```python
from build123d import *

# Parameters (mm, degrees)
BOSS_EXTRU_1_DEPTH      = 5.5
ESQUISSE6_W             = 12
ESQUISSE6_H             = 12
BOSS_EXTRU_4_DEPTH      = 4
ESQUISSE7_R             = 1.75
BOSS_EXTRU_7_DEPTH      = 0.5
ESQUISSE8_R             = 1.5
BOSS_EXTRU_9_DEPTH      = 5
CONG_1_R                = 1
CONG_2_R                = 1
CONG_3_R                = 1
ESQUISSE9_W             = 2
ESQUISSE9_H             = 11.5
ENL_V_MAT_EXTRU_1_DEPTH = 12


with BuildPart() as part:
    # Esquisse1 → Boss.-Extru.1 (new body)
    with BuildSketch(Plane.XY):
        with BuildLine():
            ThreePointArc((25, 12), (28.535533906, 10.535533906), (30, 7))
            Line((30, 7), (30, 5))
            ThreePointArc((30, 5), (28.535533906, 1.464466094), (25, 0))
            Line((25, 0), (0, 0))
            Line((0, 0), (0, 12))
            Line((0, 12), (25, 12))
        make_face()
    extrude(amount=BOSS_EXTRU_1_DEPTH)

    # Esquisse6 → Boss.-Extru.4 (add)
    with BuildSketch(Plane.XY.offset(0.75)):
        with Locations((-6, 6)):
            Rectangle(ESQUISSE6_W, ESQUISSE6_H)
    extrude(amount=BOSS_EXTRU_4_DEPTH)

    # Esquisse7 → Boss.-Extru.7 (add)
    with BuildSketch(Plane(origin=(30, 0, 0), x_dir=(0, 0, -1), z_dir=(1, 0, 0))):
        with Locations(Location((-2.75, 6, 0), (0, 0, 214.849904579))):
            Circle(ESQUISSE7_R)
    extrude(amount=BOSS_EXTRU_7_DEPTH)

    # Esquisse8 → Boss.-Extru.9 (add)
    with BuildSketch(Plane(origin=(30.5, 0, 0), x_dir=(0, 0, -1), z_dir=(1, 0, 0))):
        with Locations((-2.75, 6)):
            Circle(ESQUISSE8_R)
    extrude(amount=BOSS_EXTRU_9_DEPTH)

    # Congé1
    cong_1_edges = [part.edges().sort_by_distance(p)[0] for p in [
        (12.5, 0, 5.5),
        (28.535533906, 1.464466094, 5.5),
        (30, 6, 5.5),
        (28.535533906, 10.535533906, 5.5),
        (12.5, 12, 5.5),
    ]]
    fillet(cong_1_edges, radius=CONG_1_R - 0.0001)  # a hair under: the kernel refuses the full size

    # Congé2
    cong_2_edges = [part.edges().sort_by_distance(p)[0] for p in [
        (-12, 6, 0.75),
    ]]
    fillet(cong_2_edges, radius=CONG_2_R)

    # Congé3
    cong_3_edges = [part.edges().sort_by_distance(p)[0] for p in [
        (12.5, 0, 0),
        (28.535533906, 1.464466094, 0),
        (30, 6, 0),
        (28.535533906, 10.535533906, 0),
        (12.5, 12, 0),
    ]]
    fillet(cong_3_edges, radius=CONG_3_R - 0.0001)  # a hair under: the kernel refuses the full size

    # Esquisse9 → Enlèv. mat.-Extru.1 (cut)
    with BuildSketch(Plane.ZY.offset(12)):
        with Locations((3.25, 6)):
            Rectangle(ESQUISSE9_W, ESQUISSE9_H)
    extrude(amount=-ENL_V_MAT_EXTRU_1_DEPTH, mode=Mode.SUBTRACT)


solid = part.part
```
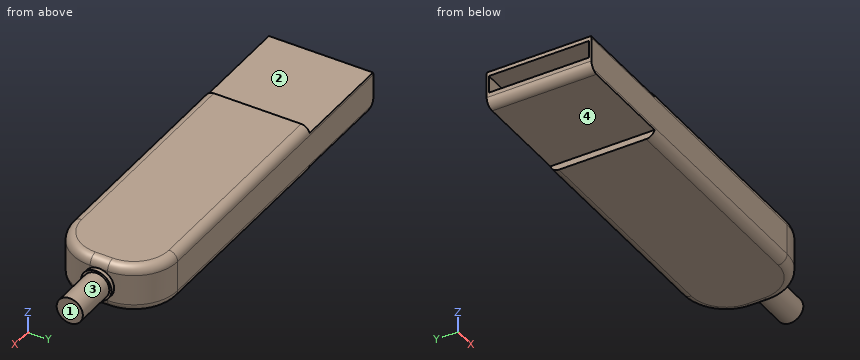
The listing builds one solid part. Answer for the finished solid, in the listing's coordinates (mm). Face numbers are marked on the shaded views. A direction names the side the tool comes from. Coordinates: 2 decimals unless noted, no trailing zeros. Loops run counter-clockwise (first coordinate to the right, second up) from the corner with the lowest first, then second, coordinate; pieces in that order, holes last. Notation, with made-up numbers: (68.25, 6) -> (110.25, 6) arc R18 ccw to (110.25, 31) -> close; hole circle Ø8 at (-30.5, -12.5). An arc over 180 degrees is marked (long way). Use one line per item in the form item = value. Start each with the question number.
Item 1: The part is cut by section B-B on z = 2.75. Determine the outline of the cut face in (x, y), then the cut area to 3 significant figures.
Item 2: A tool of negligible diameter and unlimited length cuts with its end or side. For the marked faces 1, 2, 3 and 4, from which of +Z, -Z, +X, -X, +Y, -Y can it reach the whole face along a straight path? Write none if from no direction.
Item 3: Consider L1, parallel to Z at x = -8.5, y = 1.25; L2, parallel to X at y = 9.5, z = 5.2. Determine where each line is inside the solid, lowest interval first. Write a range as [from, to].
Item 4: The part is cut by section A-A on x = -6. Determine the outline of the cut face in (y, z).
Item 5: Flat-ended cylindrical pins translate along their axes: pin 1 Ø3.5 at (x, y) = (-7.5, 7.5) entering from -Z; pin 2 Ø2 at (y, z) = (6.5, 3.5) entering from -X; pin 3 Ø6 at (x, y) = (-3.5, 6.5) entering from +Z. Find the tip coordinate at first contact, or state that the pin passes through.
Answer key:
q1.outline = (-12, 0) -> (25, 0) arc R5 ccw to (30, 5) -> (30, 4.25) -> (30.5, 4.25) -> (30.5, 4.5) -> (35.5, 4.5) -> (35.5, 7.5) -> (30.5, 7.5) -> (30.5, 7.75) -> (30, 7.75) -> (30, 7) arc R5 ccw to (25, 12) -> (-12, 12) -> (-12, 11.75) -> (0, 11.75) -> (0, 0.25) -> (-12, 0.25) -> close
q1.area = 372 mm2
q2.face_1 = +Z, -Z, +X, +Y, -Y
q2.face_2 = +Z, -X, +Y, -Y
q2.face_3 = +X
q2.face_4 = -Z, -X, +Y, -Y
q3.L1 = [0.75, 2.25], [4.25, 4.75]
q3.L2 = [0, 29]
q4.outline = (0, 1) arc R1 ccw to (0.03, 0.75) -> (11.97, 0.75) arc R1 ccw to (12, 1) -> (12, 4.5) arc R1 ccw to (11.97, 4.75) -> (0.03, 4.75) arc R1 ccw to (0, 4.5) -> close; hole (0.25, 2.25) -> (11.75, 2.25) -> (11.75, 4.25) -> (0.25, 4.25) -> close
q5.pin_1 = 0.75
q5.pin_2 = -12
q5.pin_3 = 4.75
